from build123d import *

# Parameters (mm, degrees)
SKETCH1_R           = 191
BOSS_EXTRUDE1_DEPTH = 4
M6_TAPPED_HOLE1_D   = 5
CIRPATTERN1_COUNT   = 10


with BuildPart() as part:
    # Sketch1 → Boss-Extrude1 (new body)
    with BuildSketch(Plane.XY):
        Circle(SKETCH1_R)
        with BuildLine():
            Line((-35, 171.464281995), (35, 171.464281995))
            ThreePointArc((35, 171.464281995), (0, -175), (-35, 171.464281995))
        make_face(mode=Mode.SUBTRACT)
    extrude(amount=BOSS_EXTRUDE1_DEPTH)

    # M6 Tapped Hole1 (through all)
    with Locations(Plane.XY.offset(4)):
        with Locations((0, 183)):
            m6_tapped_hole1 = Hole(M6_TAPPED_HOLE1_D / 2)

    # CirPattern1: M6 Tapped Hole1 ×10 about axis
    cirpattern1_axis = Axis((0, 0, 0), (0, 0, 1))
    for i in range(1, CIRPATTERN1_COUNT):
        add(m6_tapped_hole1.rotate(cirpattern1_axis, i * 360 / CIRPATTERN1_COUNT), mode=Mode.SUBTRACT)


solid = part.part
Design review of the part built by this model. Coordinates are the model's own, in mm. Coordinates: 2 decimals unless noted, no trailing zeros. Loops run counter-clockwise (first coordinate to the right, second up) from the corner with the lowest first, then second, coordinate; pieces in that order, holes last. Notation, with made-up numbers: (-14, -10.75) -> (18, -10.75) arc R24 cw to (18, 14.25) -> close; hole circle Ø11 at (-31, 16). An arc over 180 degrees is marked (long way). Use a Markdown table: item, result. Add a question column.
Item 1: We need section B-B, the plane x = -22. Write out the cut boundary in (y, z), and give its area (3 significant figures).
Item 2: The part is to be moulded in two halves that separate along Y. For faces 1 (the flat face through (84, -155, 0)), 2 (the cylindrical face through (-41.405, -186.458, 1.972)), 3 (the cylindrical face through (7.2, -174.85, 1.97)), say which applies: +Y half, -Y half, draft (parallel to the pull), parting line (faces both ways), or undercut.
Item 3: Clearance check with flat-ended pins moving along their axes: P1, Ø4, axis at x = -174.04, y = 56.55, coming from the -Z side; P2, Ø1, axis at x = 60.5, z = 3, coming from the -Y side; P3, Ø6, axis at x = 107.56, y = 148.05, coming from the -Z side; P4, Ø2, axis at x = 16, z = 1.5, coming from the -Y side. State where each tip first meets the part, or that it passes through.
Item 4: We need section A-A, the plane y = 0. Write out the cut boundary in (x, z).
Item 5: We need section C-C, the plane z = 3.2. Count the separate pieces of the cut face and the enclosed holes in it, and give its area (3 significant figures).
Item 6: Wall thickness on L1, parallel to Y at x = 48.5, z = 2.7; L2, parallel to Y at x = -117, z = 1.5; L3, parallel to X at y = 160.5, z = 2.4: over which ranges is each line inside the solid? List them lowest first. Write a range as from..to.
Numbers:
| question | item | result |
|---|---|---|
| 1 | outline | (-189.73, 0) -> (-173.61, 0) -> (-173.61, 4) -> (-189.73, 4) -> close; (171.46, 0) -> (189.73, 0) -> (189.73, 4) -> (171.46, 4) -> close |
| 1 | area | 138 mm^2 |
| 2 | face 1 | draft |
| 2 | face 2 | parting line |
| 2 | face 3 | undercut |
| 3 | P1 | passes through |
| 3 | P2 | stops at y = -181.33 |
| 3 | P3 | stops at z = 0 |
| 3 | P4 | stops at y = -190.41 |
| 4 | outline | (-191, 0) -> (-175, 0) -> (-175, 4) -> (-191, 4) -> close; (175, 0) -> (191, 0) -> (191, 4) -> (175, 4) -> close |
| 5 | separate pieces | 1 |
| 5 | enclosed holes | 11 |
| 5 | area | 18,400 mm^2 |
| 6 | L1 | y = -184.74..-168.15, 168.15..184.74 |
| 6 | L2 | y = -150.97..-130.14, 130.14..150.97 |
| 6 | L3 | x = -103.54..-69.75, 69.75..103.54 |
